Autodesk Fusion 360 part; units mm, degrees
sketch "MK3-front-plate" plane through (0, 0, 0) normal (0, 1, 0) x (1, 0, 0)
  line L0 (-64, 0) -> (-95, 0)
  line L1 (-95, 0) -> (-102.5, -7)
  line L2 (-102.5, -7) -> (-102.5, -33)
  line L3 (-102.5, -33) -> (-92.5, -50)
  line L4 (-92.5, -50) -> (92.5, -50)
  line L5 (102.5, -33) -> (102.5, -7)
  line L6 (64, 0) -> (52, -11.5)
  line L7 (102.5, -7) -> (95, 0)
  line L8 (-52, -11.5) -> (-64, 0)
  line L9 (95, 0) -> (64, 0)
  line L10 (52, -11.5) -> (-52, -11.5)
  line L11 (92.5, -50) -> (102.5, -33)
  line L12 (-64, 0) -> (64, 0) construction
  line L13 (-73.4, 0) -> (-73.4, -50) construction
  line L14 (-96.6, 0) -> (-96.6, -50) construction
  circle A0 centre (-73.4, -9.9) radius 2.5
  circle A1 centre (-96.6, -9.9) radius 2.5
  circle A2 centre (-73.4, -33.1) radius 2.5
  circle A3 centre (-96.6, -33.1) radius 2.5
  line L15 (-96.6, -40) -> (-73.4, -40) construction
  circle A4 centre (-90.5, -40) radius 1.5
  circle A5 centre (-79.5, -40) radius 1.5
  circle A6 centre (0, -46) radius 1.5
  line L16 (0, 0) -> (0, -50) construction
  circle A7 centre (0, -20) radius 1.5
  line L17 (-60, -21) -> (-60, -32) construction
  circle A8 centre (-60, -21) radius 1.65
  circle A9 centre (-60, -32) radius 1.65
  circle A10 centre (60, -32) radius 1.65
  circle A11 centre (60, -21) radius 1.65
  circle A12 centre (73.4, -9.9) radius 2.5
  circle A13 centre (96.6, -9.9) radius 2.5
  circle A14 centre (96.6, -33.1) radius 2.5
  circle A15 centre (73.4, -33.1) radius 2.5
  circle A16 centre (79.5, -40) radius 1.5
  circle A17 centre (90.5, -40) radius 1.5
  line L18 (0, -33.1) -> (-102.5, -33.1) construction
  line L19 (-102.5, -9.9) -> (0, -9.9) construction
  dimension "d3" = 50
  dimension "d4" = 205
  dimension "d5" = 7.5
  dimension "d12" = 10
  dimension "d16" = 17
  dimension "d26" = 5
  dimension "d27" = 5
  dimension "d28" = 5
  dimension "d29" = 5
  dimension "d37" = 3
  dimension "d40" = 3
  dimension "d46" = 4
  dimension "d48" = 3
  dimension "d49" = 3
  dimension "d50" = 10
  dimension "d51" = 16.9
  dimension "d52" = 3.3
  dimension "d53" = 3.3
  dimension "d54" = 18
  dimension "d56" = 42.5
  dimension "d57" = 5.9
  dimension "d58" = 29.1
  dimension "d59" = 40.1
  dimension "d60" = 102.5
  dimension "d61" = 43
  dimension "d62" = 29
  dimension "d63" = 12
  dimension "d64" = 23
  dimension "d65" = 50.5
  dimension "d66" = 12
  dimension "d67" = 38.5
  dimension "d68" = 30
extrude "Extrude1" add sketch "MK3-front-plate" along normal blind 4
Geometry check sheet. Reference: the model listing, model coordinates, mm. A direction names the side the tool comes from. Coordinates: 2 decimals unless noted, no trailing zeros. Order: outer loops, then holes, each group sorted by start corner. A loop starts at its lowest first (then second) coordinate and runs counter-clockwise, first axis right, second up.
Item 1: Scan lines: line 1 along Z through (x, y) = (-73.4, 1.85); line 2 along Z through (x, y) = (90.5, 1.2); line 3 along X through (y, z) = (2.5, 21). Record each from-to range of solid material in increasing order.
Item 2: Tool access check on faces 1 (the flat face through (58.084, 1.972, 5.669)), 2 (the flat face through (-98.698, 1.972, 3.451)). Record the directions out of +Z, -Z, +X, -X, +Y, -Y that give a thin tool (end or side, any length) a straight path to the whole face; none if there is none.
Item 3: Mould release check, pull along Z, two halves, no side actions. Record for faces 3 (the flat face through (1, 2, 11.5)), 4 (the cylindrical face through (-61.216, 1.972, 33.115)), 5 (the flat face through (-1, 2, 50)), 6 (the cylindrical face through (71.4, 2, 31.6)): released by +Z, released by -Z, zero draft, split by the parting line, or undercut.
Item 4: Section check A-A (x = 73.4). Enter the section's corners in (y, z), plus the area to 3 significant figures.
Item 5: Depth check by flat-ended pin: pin 1 (3 mm diameter, centred on x = 60, z = 32, fed in from +Y). Enter the tip coordinate at first touch or a pass-through.
Item 6: Section check C-C (x = -32). Enter the section's corners in (y, z), plus the area to 3 significant figures.
Item 7: Section check B-B (y = 2.4). Count the separate pieces of the cut face and the enclosed holes in it, plus the area to 3 significant figures.
Check sheet entries:
1. line 1: z = 0 to 7.4, 12.4 to 30.6, 35.6 to 50
1. line 2: z = 0 to 38.5, 41.5 to 50
1. line 3: x = -102.5 to -61.65, -58.35 to -1.12, 1.12 to 58.35, 61.65 to 102.5
2. face 1: -Z, +Y, -Y
2. face 2: -Z, -X, +Y, -Y
3. face 3: released by -Z
3. face 4: undercut
3. face 5: released by +Z
3. face 6: undercut
4. outline: (0, 0) - (4, 0) - (4, 7.4) - (0, 7.4) - close; (0, 12.4) - (4, 12.4) - (4, 30.6) - (0, 30.6) - close; (0, 35.6) - (4, 35.6) - (4, 50) - (0, 50) - close
4. area: 160 mm2
5. pin 1: passes through
6. outline: (0, 11.5) - (4, 11.5) - (4, 50) - (0, 50) - close
6. area: 154 mm2
7. separate pieces: 1
7. enclosed holes: 18
7. area: 8,460 mm2
